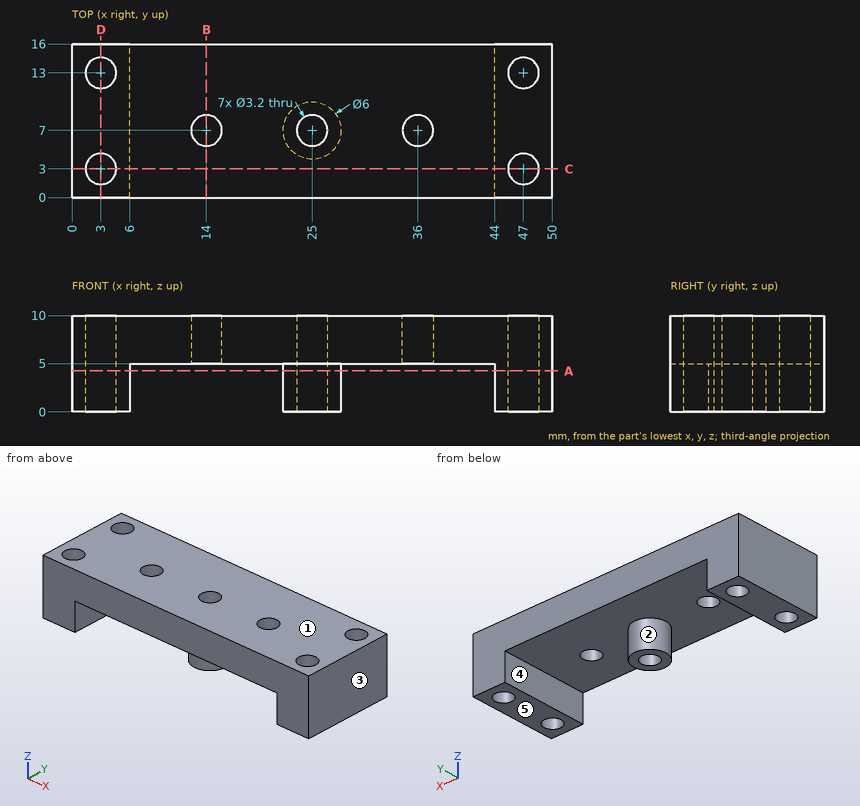
Drawing for the job (mm, zero at the part's lowest x, y, z). A direction names the side the tool comes from. Give positions to 0.01 mm unless a question says otherwise; leave off trailing zeros. Loops run counter-clockwise (first coordinate to the right, second up) from the corner with the lowest first, then second, coordinate; pieces in that order, holes last. Notation, with made-up numbers: M 88,-2.5 L 108,-2.5 A14 cw 108,3.5 Z; hole C 17,65 d8. An arc over 180 degrees is marked long. One line per question, with ' | ' between items. Start each with the question number.
1. Two-plate mould, pull along X, no slides. Class the marked faces 1, 2 and 3: pulls with the +X half, pulls with the -X half, needs draft (parallel to the pull), parting line crosses it, or undercut.
2. 3-axis set-ups, long thin cutter, end or side, ignore diameter. For the marked faces 4 and 5: which of +Z, -Z, +X, -X, +Y, -Y reach the whole face in a straight line?
3. Saw through at B-B on x = 14. Give the cut face in (y, z).
4. Saw through at D-D on x = 3. Give the cut face in (y, z), plus the area to 3 significant figures.
5. Flat gauge pin, fed straight in: pin 1 (3 mm diameter, centred on x = 28.5, z = 1, fed in from +Y). Where does the tip first touch, or does it go through?
6. Saw through at A-A on z = 4.25. Give the cut face in (x, y).
7. Probe L1, parallel to Y at x = 3, z = 6.5; L2, parallel to Y at x = 14, z = 8.45; L3, parallel to X at y = 13.25, z = 6.5. List the from-to ranges inside material, lowest first. Write a range as from..to.
8. Saw through at C-C on y = 3. Give the cut face in (x, z), plus the area to 3 significant figures.
Result sheet:
1) face 1: needs draft | face 2: undercut | face 3: pulls with the +X half
2) face 4: -Z, +Y, -Y | face 5: -Z, +X, -X, +Y, -Y
3) outline: M 0,5 L 5.4,5 L 5.4,10 L 0,10 Z; M 8.6,5 L 16,5 L 16,10 L 8.6,10 Z
4) outline: M 0,0 L 1.4,0 L 1.4,10 L 0,10 Z; M 4.6,0 L 11.4,0 L 11.4,10 L 4.6,10 Z; M 14.6,0 L 16,0 L 16,10 L 14.6,10 Z | area: 96.0 mm^2
5) pin 1: stops at y = 9.24
6) outline: M 0,0 L 6,0 L 6,16 L 0,16 Z; C 25,7 d6; M 44,0 L 50,0 L 50,16 L 44,16 Z; hole C 3,3 d3.2; hole C 3,13 d3.2; hole C 25,7 d3.2; hole C 47,3 d3.2; hole C 47,13 d3.2
7) L1: y = 0..1.4, 4.6..11.4, 14.6..16 | L2: y = 0..5.4, 8.6..16 | L3: x = 0..1.42, 4.58..45.42, 48.58..50
8) outline: M 0,0 L 1.4,0 L 1.4,10 L 0,10 Z; M 4.6,0 L 6,0 L 6,5 L 44,5 L 44,0 L 45.4,0 L 45.4,10 L 4.6,10 Z; M 48.6,0 L 50,0 L 50,10 L 48.6,10 Z | area: 246 mm^2
